Can you work these out from the model? Positions are in its coordinate system, mm. A direction names the side the tool comes from. Round coordinates to 2 decimals unless told otherwise and drop trailing zeros.
```python
from build123d import *


with BuildPart() as f1:
    # F0 (on Top) → F1 (revolve)
    with BuildSketch(Plane.XY):
        Polygon((39.014403, 22.7076), (0, 46.177197), (0, -34.8996), (18.288001, -34.8996), (18.288001, -16.6116), (37.490401, -16.6116), (18.288001, 4.4196), (39.014403, 4.4196), (18.288001, 22.7076), align=None)
    revolve(axis=Axis((0, 2.743199, 0), (0, -1, 0)))


solid = f1.part
```
(1) Which directions (+Z, -Z, +X, -X, +Y, -Y) give clear straight access to the entire face, cutting with the end or side of a thin tool? Please do faces 1 (the conical face through (18.33, 3.4, 5.77)), 2 (the flat face through (-8, -16.612, 17)), 3 (the flat face through (0, -34.9, 0)).
(2) If I drill on line 1 (Y direction, x = 27, z = -19); line 2 (Y direction, x = 17.5, z = 12); line 3 (Z direction, x = 6, y = -23.5), over which ranges is the centre line in solid material (lowest first)?
(3) For pin 1 (1 mm diameter, centred on x = -15, y = 21.5, fed in from +Z); pin 2 (6 mm diameter, centred on y = -19, z = -24.5, fed in from -X); pin 3 (1.5 mm diameter, centred on y = 23, z = 21.5, fed in from -X); pin 4 (3 mm diameter, centred on x = -21, y = -18.5, fed in from +Z), each with a flat end and sliding along its axis, tell me the tip position at first contact or that it passes through.
(4) Suppose I cut it at A-A (x = 34). Give the number of separate pieces and of enclosed holes in the cut face, then the cut area to 3 significant figures.
Check result:
1. face 1: none
1. face 2: -Y
1. face 3: +Z, -Z, +X, -X, -Y
2. line 1: y = -16.61 to -11.71, 4.42 to 9.71, 22.71 to 26.32
2. line 2: y = -16.61 to 1.21, 4.42 to 20.12, 22.71 to 33.41
2. line 3: z = -17.28 to 17.28
3. pin 1: stops at z = 13.73
3. pin 2: stops at x = -29.85
3. pin 3: stops at x = -33
3. pin 4: passes through
4. separate pieces: 3
4. enclosed holes: 0
4. area: 267 mm2
